```python
from build123d import *

# Parameters (mm, degrees)
SKETCH1_W               = 37
SKETCH1_H               = 37
BOSS_EXTRUDE1_DEPTH     = 34
CUT_EXTRUDE1_DEPTH      = 20
CUT_EXTRUDE1_DEPTH_BACK = 20
SKETCH2_R               = 31.75
SKETCH5_R               = 16
CUT_EXTRUDE2_DEPTH      = 43.901048938
SKETCH6_R               = 2
CUT_EXTRUDE3_DEPTH      = 28.41687798


with BuildPart() as part:
    # Sketch1 → Boss-Extrude1 (new body)
    with BuildSketch(Plane.XY):
        Rectangle(SKETCH1_W, SKETCH1_H)
    extrude(amount=BOSS_EXTRUDE1_DEPTH)

    # Sketch2 → Cut-Extrude1 (cut, two sides: drawn at the far end of the back side and taken through both)
    with BuildSketch(Plane(origin=(0, 0, 0), x_dir=(0, 0, -1), z_dir=(1, 0, 0)).offset(-CUT_EXTRUDE1_DEPTH_BACK)):
        Circle(SKETCH2_R)
    extrude(amount=CUT_EXTRUDE1_DEPTH + CUT_EXTRUDE1_DEPTH_BACK, mode=Mode.SUBTRACT)

    # Sketch5 → Cut-Extrude2 (cut, through all)
    with BuildSketch(Plane.XY):
        with Locations(Location((0, 0, 0), (0, 0, 180))):
            Circle(SKETCH5_R)
    extrude(amount=CUT_EXTRUDE2_DEPTH, mode=Mode.SUBTRACT)

    # Sketch6 → Cut-Extrude3 (cut, through all)
    with BuildSketch(Plane.XY.offset(34)):
        with Locations((-14.610912703, -14.610912703)):
            Circle(SKETCH6_R)
        with Locations((14.610912703, -14.610912703)):
            Circle(SKETCH6_R)
        with Locations((14.610912703, 14.610912703)):
            Circle(SKETCH6_R)
        with Locations((-14.610912703, 14.610912703)):
            Circle(SKETCH6_R)
    extrude(amount=-CUT_EXTRUDE3_DEPTH, mode=Mode.SUBTRACT)


solid = part.part
```
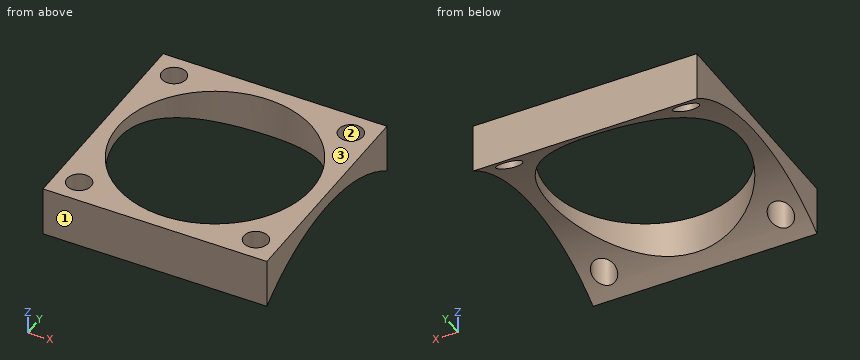
Here's how the part is built. I have some questions about the finished solid (model axes, mm). Face numbers are marked on the shaded views. Round coordinates to 2 decimals unless told otherwise and drop trailing zeros. Order: outer loops, then holes, each group sorted by start corner. A loop starts at its lowest first (then second) coordinate and runs counter-clockwise, first axis right, second up. Notation, with made-up numbers: M 51.5,89 L 64.5,89 A26 cw 64.5,123 Z; hole C 62.5,-38 d10. An arc over 180 degrees is marked long. Answer as CSV lines item,"result".
Item 1: Imagine slicing it at D-D on x = 15.5. List the corners of the cut face in (y, z) for me, and give its area (3 significant figures).
From the geometry:
outline,"M -18.5,25.8 A31.75 cw -16.4,27.18 L -16.4,34 L -18.5,34 Z; M -12.82,29.05 A31.75 cw -3.97,31.5 L -3.97,34 L -12.82,34 Z; M 3.97,31.5 A31.75 cw 12.82,29.05 L 12.82,34 L 3.97,34 Z; M 16.4,27.18 A31.75 cw 18.5,25.8 L 18.5,34 L 16.4,34 Z"
area,"93.3 mm2"
Item 2: Please list where these lines run through material, in increasing order: L1, parallel to X at y = -13.5, z = 30.5; L2, parallel to Y at x = 0, z = 32; L3, parallel to X at y = 14, z = 32. Write a range as [from, to].
From the geometry:
L1,"[-18.5, -16.27], [-12.95, -8.59], [8.59, 12.95], [16.27, 18.5]"
L2,"[-18.5, -16], [16, 18.5]"
L3,"[-18.5, -16.52], [-12.71, -7.75], [7.75, 12.71], [16.52, 18.5]"
Item 3: Imagine slicing it at B-B on x = 0. List the corners of the cut face in (y, z) for me, and give its area (3 significant figures).
From the geometry:
outline,"M -18.5,25.8 A31.75 cw -16,27.42 L -16,34 L -18.5,34 Z; M 16,27.42 A31.75 cw 18.5,25.8 L 18.5,34 L 16,34 Z"
area,"36.8 mm2"
Item 4: Imagine slicing it at A-A on z = 29.5. List the corners of the cut face in (x, y) for me, and give its area (3 significant figures).
From the geometry:
outline,"M -18.5,-18.5 L 18.5,-18.5 L 18.5,-11.74 L 10.87,-11.74 A16 cw -10.87,-11.74 L -18.5,-11.74 Z; M -18.5,11.74 L -10.87,11.74 A16 cw 10.87,11.74 L 18.5,11.74 L 18.5,18.5 L -18.5,18.5 Z; hole C -14.61,-14.61 d4; hole C -14.61,14.61 d4; hole C 14.61,-14.61 d4; hole C 14.61,14.61 d4"
area,"323 mm2"
Item 5: We'd pull the mould along Y, two halves only. Please class the marked faces 1, 2 and 3: +Y half, -Y half, draft (parallel to the pull), parting line (faces both ways), or undercut.
From the geometry:
face 1,"-Y half"
face 2,"undercut"
face 3,"draft"
Item 6: Imagine slicing it at C-C on y = 0. List the corners of the cut face in (x, z) for me, and give its area (4 significant figures).
From the geometry:
outline,"M -18.5,31.75 L -16,31.75 L -16,34 L -18.5,34 Z; M 16,31.75 L 18.5,31.75 L 18.5,34 L 16,34 Z"
area,"11.25 mm2"
